```python
from build123d import *

# Parameters (mm, degrees)
SKETCH_1_W             = 36
SKETCH_1_H             = 89.64
SM_BASE_FLANGE_1_DEPTH = 3
OTHER_START            = -18
OTHER_1_DEPTH          = 36
OTHER_1_2_DEPTH        = 36
SKETCH_7_R             = 14
SKETCH_7_R_2           = 1.8
CUT_EXTRUDE_1_DEPTH    = 10
CHAMFER_1_SIZE         = 3
SKETCH_8_R             = 2.75
CUT_EXTRUDE_2_DEPTH    = 10


# Read off the part's stored shape, not the designer's step: Нарисованный сгиб1
# Sheet-metal steps are written as plain solids
with BuildPart() as part:
    # Sketch 1 → Базовая кромка1 (new body)
    with BuildSketch(Plane(origin=(0, 0, 0), x_dir=(1, 0, 0), z_dir=(0, 1, 0))):
        Rectangle(SKETCH_1_W, SKETCH_1_H)
    extrude(amount=-SM_BASE_FLANGE_1_DEPTH)

    # Other 1 outline → Other 1 (cut)
    with BuildSketch(Plane.YZ.offset(OTHER_START)):
        with BuildLine():
            Line((0, -44.82), (0, 6.075437354))
            ThreePointArc((0, 6.075437354), (-2.204836823, 8.579629651), (-3, 11.82))
            Line((-3, 11.82), (-3, -44.82))
            Line((-3, -44.82), (0, -44.82))
        make_face()
    extrude(amount=OTHER_1_DEPTH, mode=Mode.SUBTRACT)

    # Other 1 2 outline → Other 1 2 (add)
    with BuildSketch(Plane.YZ.offset(OTHER_START)):
        with BuildLine():
            Line((52.000620203, 7.82), (4, 7.82))
            ThreePointArc((4, 7.82), (1.171572875, 8.991572875), (0, 11.82))
            Line((0, 11.82), (0, 6.075437354))
            ThreePointArc((0, 6.075437354), (1.903805654, 5.141229959), (4, 4.82))
            Line((4, 4.82), (52.000620203, 4.82))
            Line((52.000620203, 4.82), (52.000620203, 7.82))
        make_face()
    extrude(amount=OTHER_1_2_DEPTH)

    # Эскиз7 → Вырез-Вытянуть1 (cut)
    with BuildSketch(Plane.XY.offset(7.82)):
        with Locations((0, 34.000620203)):
            Circle(SKETCH_7_R)
        with Locations((13, 47.000620203)):
            Circle(SKETCH_7_R_2)
        with Locations(Location((-13, 47.000620203, 0), (0, 0, 90))):
            Circle(SKETCH_7_R_2)
        with Locations((-13, 21.000620203)):
            Circle(SKETCH_7_R_2)
        with Locations(Location((13, 21.000620203, 0), (0, 0, 90))):
            Circle(SKETCH_7_R_2)
    extrude(amount=-CUT_EXTRUDE_1_DEPTH, mode=Mode.SUBTRACT)

    # Фаска1
    chamfer_1_edges = [part.edges().sort_by_distance(p)[0] for p in [
        (18, -1.5, 44.82),
        (-18, -1.5, 44.82),
        (-18, 52.000620203, 6.32),
        (18, 52.000620203, 6.32),
    ]]
    chamfer(chamfer_1_edges, length=CHAMFER_1_SIZE)

    # Эскиз8 → Вырез-Вытянуть2 (cut)
    with BuildSketch(Plane(origin=(0, 0, 0), x_dir=(1, 0, 0), z_dir=(0, 1, 0))):
        with Locations(Location((-10, -29.82, 0), (0, 0, 270))):
            Circle(SKETCH_8_R)
        with Locations(Location((10, -29.82, 0), (0, 0, 90))):
            Circle(SKETCH_8_R)
    extrude(amount=-CUT_EXTRUDE_2_DEPTH, mode=Mode.SUBTRACT)


solid = part.part
```
Geometry check sheet. Reference: the model listing, model coordinates, mm. A direction names the side the tool comes from. Round coordinates to 2 decimals unless told otherwise and drop trailing zeros. Write each loop counter-clockwise with the first axis right and the second up, starting at its lowest first coordinate (ties: lowest second). Pieces come first, ordered by that corner, then holes. Notation, with made-up numbers: (40.5, -27.75) -> (99.5, -27.75) arc R35 ccw to (99.5, 10.25) -> close; hole circle Ø2 at (-35.5, 4). An arc over 180 degrees is marked (long way). Put each result on its own line as item: value.
1) Depth check by flat-ended pin: P1, Ø4, axis at x = 13, y = 21, coming from the +Z side; P2, Ø9, axis at x = -10, z = 29.82, coming from the +Y side. Enter the tip coordinate at first touch or a pass-through.
Recorded:
P1: stops at z = 7.82
P2: stops at y = 0
2) Release check for a two-part mould opening along Z. For faces 1 (the face through (12.766, 48.785, 6.341)), 2 (the face through (-16.48, -1.48, 43.34)), 3 (the face through (9.17, -1.48, 27.2)), 4 (the face through (-9.17, -1.48, 32.44)) record: pulls with the +Z half, pulls with the -Z half, needs draft (parallel to the pull), parting line crosses it, or undercut.
Recorded:
face 1: needs draft
face 2: pulls with the +Z half
face 3: undercut
face 4: undercut
3) Thickness scan on probe 1 along Z at (x, y) = (-13.5, 13.5); probe 2 along Y at (x, z) = (-10, 35); probe 3 along Y at (x, z) = (0, 6). Record the ranges inside material, lowest first. Write a range as from..to.
Recorded:
probe 1: z = 4.82..7.82
probe 2: y = -3..0
probe 3: y = 0.11..20, 48..52
4) Cross-section at A-A, the plane z = 29.82. Enter the section's corners in (x, y).
Recorded:
outline: (-18, -3) -> (-12.75, -3) -> (-12.75, 0) -> (-18, 0) -> close; (-7.25, -3) -> (7.25, -3) -> (7.25, 0) -> (-7.25, 0) -> close; (12.75, -3) -> (18, -3) -> (18, 0) -> (12.75, 0) -> close
5) Access from +Z, -Z, +X, -X, +Y, -Y to the whole of each face (thin tool, end or side, straight path). Record for faces 5 (the face through (0, 18, 7.82)), 6 (the face through (18, 11, 7)).
Recorded:
face 5: +Z, +X, -X, +Y
face 6: +Z, -Z, +X, +Y, -Y
6) Cross-section at D-D, the plane x = 10. Enter the section's corners in (y, z).
Recorded:
outline: (-3, 11.82) arc R7 ccw to (4, 4.82) -> (24.2, 4.82) -> (24.2, 7.82) -> (4, 7.82) arc R4 cw to (0, 11.82) -> (0, 27.07) -> (-3, 27.07) -> close; (-3, 32.57) -> (0, 32.57) -> (0, 44.82) -> (-3, 44.82) -> close; (43.8, 4.82) -> (52, 4.82) -> (52, 7.82) -> (43.8, 7.82) -> close
7) Cross-section at C-C, the plane y = 35.5. Enter the section's corners in (x, z), plus the area to 3 significant figures.
Recorded:
outline: (-18, 4.82) -> (-13.92, 4.82) -> (-13.92, 7.82) -> (-18, 7.82) -> close; (13.92, 4.82) -> (18, 4.82) -> (18, 7.82) -> (13.92, 7.82) -> close
area: 24.5 mm2
8) Cross-section at B-B, the plane x = 0. Enter the section's corners in (y, z).
Recorded:
outline: (-3, 11.82) arc R7 ccw to (4, 4.82) -> (20, 4.82) -> (20, 7.82) -> (4, 7.82) arc R4 cw to (0, 11.82) -> (0, 44.82) -> (-3, 44.82) -> close; (48, 4.82) -> (52, 4.82) -> (52, 7.82) -> (48, 7.82) -> close
